Could you check a few things on this model? Use its own coordinates, in mm. Face numbers are marked on the shaded views. Give positions to 0.01 mm unless a question says otherwise; leave off trailing zeros. Loops run counter-clockwise (first coordinate to the right, second up) from the corner with the lowest first, then second, coordinate; pieces in that order, holes last. Notation, with made-up numbers: (49.5, -16.5) - (104.5, -16.5) arc R14 ccw to (104.5, -6.5) - close; hole circle Ø4 at (49, 64). An arc over 180 degrees is marked (long way). Write each question's results on one line, items separated by ' | '. Start each with the question number.
1) If we mould it in two halves opening along X, with no side actions, what happens to the marked faces 1, 2 and 3? For each: +X half, -X half, draft (parallel to the pull), parting line (faces both ways), or undercut.
2) I'm going to push flat-ended pins straight in: pin 1 (10 mm diameter, centred on y = -50.5, z = 12.5, fed in from +X); pin 2 (12 mm diameter, centred on x = 7, y = -113.5, fed in from +Z); pin 3 (1 mm diameter, centred on y = -58.5, z = -18, fed in from +X). Where does each tip first touch, or does it pass through?
3) I want a section at A-A, the plane y = -113.5. Write out the boundary of the cut face in (x, z), and give its area (3 significant figures).
4) If I drill on probe 1 along Y at (x, z) = (-11, -2) (3 decimals); probe 2 along Z at (x, y) = (-8, -142.5), over which ranges is the centre line in solid material (lowest first)? Write a range as [from, to].
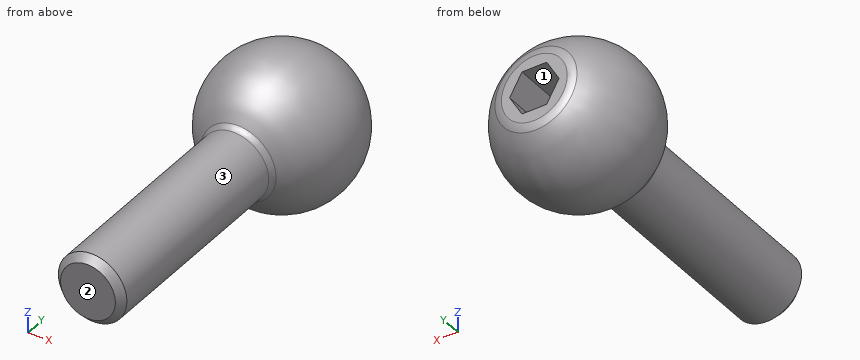
Autodesk Inventor part; units mm, degrees
ref_plane "Work Plane1" through (0, 0, 0) normal (0, 1, 0) x (-1, 0, 0)
ref_plane "Work Plane2" through (2.0638, 3.5745, 0) normal (0, 1, 0) x (-1, 0, 0)
ref_plane "YZ Plane" through (0, 0, 0) normal (1, 0, 0) x (0, 1, 0)
sketch "Sketch1" plane through (0, 0, 0) normal (0, 0, 1) x (1, 0, 0)
  line L0 (0, 9.0251) -> (0, -20.025)
  arc A0 (0, 4.1275) -> (-1.905, -3.6616) centre (0, 0) ccw
  line L1 (-1.905, -3.6616) -> (-1.905, -15.875)
  line L2 (-1.905, -15.875) -> (0, -15.875)
  dimension "d0" = 8.255
  dimension "d1" = 15.875
  dimension "d2" = 3.81
revolve "Revolution1" add sketch "Sketch1" angle 360 about axis through (0, 0, 0) along (0, -1, 0)
fillet "Fillet1" radius 0.381 1 edges at (1.905, -3.6616, 0)
chamfer "Chamfer1" distance 0.381 angle 45 1 edges at (1.905, -15.875, 0)
sketch "Sketch2" plane through (0, 0, 0) normal (0, 0, 1) x (1, 0, 0)
  line L0 (-1.524, -15.875) -> (-1.905, -15.494)
  line L1 (-1.905, -15.494) -> (-1.905, -3.886)
  arc A0 (-1.905, -3.886) -> (-2.0928, -3.5576) centre (-2.286, -3.886) ccw
  arc A1 (2.0928, -3.5576) -> (-2.0928, -3.5576) centre (0, 0) ccw
  arc A2 (2.0928, -3.5576) -> (1.905, -3.886) centre (2.286, -3.886) ccw
  line L2 (1.905, -3.886) -> (1.905, -15.494)
  line L3 (1.905, -15.494) -> (1.524, -15.875)
  line L4 (1.524, -15.875) -> (-1.524, -15.875)
  point P0 (2.0638, 3.5745)
ref_plane "Work Plane1" through (0, 0, 0) normal (0, 1, 0) x (-1, 0, 0)
ref_plane "Work Plane2" through (2.0638, 3.5745, 0) normal (0, 1, 0) x (-1, 0, 0)
split "Split1" plane through (2.0638, 3.5745, 0) removes the side toward (0, 1, 0)
fillet "Fillet2" radius 0.8128 1 edges at (2.0638, 3.5745, 0)
sketch "Sketch3" plane through (0, 3.5745, 0) normal (0, 1, 0) x (1, 0, 0)
  circle A0 centre (0, 0) radius 1.524
  line L0 (1.3748, 0) -> (0.6874, -1.1906)
  line L1 (0.6874, -1.1906) -> (-0.6874, -1.1906)
  line L2 (-0.6874, -1.1906) -> (-1.3748, 0)
  line L3 (-1.3748, 0) -> (-0.6874, 1.1906)
  line L4 (-0.6874, 1.1906) -> (0.6874, 1.1906)
  line L5 (0.6874, 1.1906) -> (1.3748, 0)
  dimension "d11" = 2.3813
extrude "Extrusion1" cut sketch "Sketch3" against normal blind 2.54 contours L0 L1 L2 L3 L4 L5
thread "Thread1"
scale "Scale1" factors (10, 10, 10) then translate (0, 0, 0) bodies 1
properties part number "Pillow Ball"
Answers:
1) face 1: undercut | face 2: draft | face 3: parting line
2) pin 1: stops at x = 17.51 | pin 2: stops at z = 19.02 | pin 3: stops at x = 7.53
3) outline: circle Ø38.1 at (0, 0) | area: 1,140 mm2
4) probe 1: y = [-158.75, 10.345] | probe 2: z = [-17.29, 17.29]
